Autodesk Inventor part; units mm, degrees
ref_plane "YZ Plane" through (0, 0, 0) normal (1, 0, 0) x (0, 1, 0)
ref_plane "XZ Plane" through (0, 0, 0) normal (0, 1, 0) x (-1, 0, 0)
ref_plane "XY Plane" through (0, 0, 0) normal (0, 0, 1) x (1, 0, 0)
sketch "Sketch1" plane through (0, 0, 0) normal (1, 0, 0) x (0, 1, 0)
  line L0 (-41.95, 491.5) -> (41.95, 491.5)
  line L1 (41.95, 491.5) -> (41.95, -491.5)
  line L2 (41.95, -491.5) -> (-41.95, -491.5)
  line L3 (-41.95, -491.5) -> (-41.95, 491.5)
  line L4 (-41.95, 491.5) -> (41.95, -491.5) construction
  line L5 (41.95, 491.5) -> (-41.95, -491.5) construction
  line L6 (-41.95, 491.5) -> (-988.2844, 456)
  line L7 (-988.2844, 456) -> (-988.2844, -456)
  line L8 (-988.2844, -456) -> (-41.95, -491.5)
  line L9 (-308.05, 481.5177) -> (-308.05, -481.5177)
  line L10 (-988.2844, 456) -> (-1098.8336, 370.0997)
  arc A0 (-988.2844, 456) -> (-1068.8274, 393.4155) centre (-985.0081, 368.664) ccw
  line L11 (-988.2844, 0) -> (-1170.4564, 0)
  line L12 (-1098.8336, 370.0997) -> (-1098.8336, 0)
  line L13 (-988.2844, -456) -> (-1098.8336, -370.0997)
  arc A1 (-1068.8274, -393.4155) -> (-988.2844, -456) centre (-985.0081, -368.664) ccw
  line L14 (-1098.8336, -370.0997) -> (-1098.8336, 0)
  point P0 (0, 0)
  point P1 (-41.95, 0)
  dimension "d0" = 983
  dimension "d1" = 83.9
  dimension "d3" = 912
  dimension "d4" = 947
  dimension "d5" = 350
  dimension "d9" = 35.7
  dimension "d10" = 102
  dimension "d11" = 38
extrude "Plate2" add sketch "Sketch1" along normal blind 1.5 contours L9 L8 L7 L6
sheet face with bend "Face3" sketch "Sketch1" thickness 1.5 toward (1, 0, 0) bend radius 1.5 contours L7 L11 L12 L10 | L10 A0 | L13 L14 L11 L7 | A1 L13
bend "Bend1"
equation "\"d7\" = Thickness"
equation "\"d12\" = BendRadius"
equation "\"d13\" = BendReliefWidth"
equation "\"d15\" = MinimumRemnant"
equation "\"d14\" = BendReliefDepth"
equation "\"d16\" = TransitionRadius"
equation "\"BendRadius\" = Thickness"
equation "\"BendReliefWidth\" = Thickness"
equation "\"BendReliefDepth\" = 0.5 * Thickness"
equation "\"CornerReliefSize\" = 4 * Thickness"
equation "\"MinimumRemnant\" = 2 * Thickness"
equation "\"TransitionRadius\" = BendRadius"
equation "\"JacobiRadiusSize\" = BendRadius"
equation "\"GapSize\" = Thickness"
properties part number "CHAPA_2" material "Steel, Mild, Welded"
Source: CAD feature listing. Evaluate the final solid. Frame: model axes, mm. Coordinates: 2 decimals unless noted, no trailing zeros. Order: outer loops, then holes, each group sorted by start corner. A loop starts at its lowest first (then second) coordinate and runs counter-clockwise, first axis right, second up. Notation, with made-up numbers: M 15,-5 L 35,-5 A14 ccw 35,10 Z; hole C 17.5,-33 d4. An arc over 180 degrees is marked long. Write each question's results on one line, items separated by ' | '. Start each with the question number.
1) Section query C-C (z = -410.5). Return the cut outline in (x, y), plus the area to 3 significant figures.
2) Line query: line 1 (Z direction, x = 1.1, y = -402.5); line 2 (Z direction, x = 0.85, y = -681.5); line 3 (Y direction, x = 0.2, z = 434.5). Output: solid intervals per line, ascending. Write a range as from..to.
3) Section query B-B (y = -721.5). Return the cut outline in (x, z).
4) Section query A-A (x = 1.2). Return the cut outline in (y, z).
Answers:
1) outline: M 0,-1061.74 L 1.5,-1061.74 L 1.5,-308.05 L 0,-308.05 Z | area: 1,130 mm^2
2) line 1: z = -477.97..477.97 | line 2: z = -467.51..467.51 | line 3: y = -1042.49..-308.05
3) outline: M 0,-466.01 L 1.5,-466.01 L 1.5,466.01 L 0,466.01 Z
4) outline: M -1098.83,-370.1 L -1068.83,-393.42 A87.4 ccw -988.28,-456 L -308.05,-481.52 L -308.05,481.52 L -988.28,456 A87.4 ccw -1068.83,393.42 L -1098.83,370.1 Z
